Input: part model. Units: mm. Frame: model coordinates. A direction names the side the tool comes from. Give positions to 0.01 mm unless a question says otherwise; leave off trailing zeros. Order: outer loops, then holes, each group sorted by start corner. A loop starts at its lowest first (then second) coordinate and runs counter-clockwise, first axis right, second up.
```python
from build123d import *

# Parameters (mm, degrees)
SKETCH1_W           = 40
SKETCH1_H           = 40
BOSS_EXTRUDE1_DEPTH = 5
SKETCH3_W           = 5
SKETCH3_H           = 40
BOSS_EXTRUDE6_DEPTH = 40
SKETCH4_R           = 2.25
CUT_EXTRUDE2_DEPTH  = 49.989794856
SKETCH5_R           = 10.5
SKETCH5_R_2         = 2
CUT_EXTRUDE3_DEPTH  = 61.415229868


with BuildPart() as part:
    # Sketch1 → Boss-Extrude1 (new body)
    with BuildSketch(Plane(origin=(0, 0, 0), x_dir=(1, 0, 0), z_dir=(0, 1, 0))):
        Rectangle(SKETCH1_W, SKETCH1_H)
    extrude(amount=BOSS_EXTRUDE1_DEPTH)

    # Sketch3 → Boss-Extrude6 (add)
    with BuildSketch(Plane(origin=(0, 5, 0), x_dir=(1, 0, 0), z_dir=(0, 1, 0))):
        with Locations((-17.5, 0)):
            Rectangle(SKETCH3_W, SKETCH3_H)
    extrude(amount=BOSS_EXTRUDE6_DEPTH)

    # Sketch4 → Cut-Extrude2 (cut, through all)
    with BuildSketch(Plane(origin=(0, 5, 0), x_dir=(1, 0, 0), z_dir=(0, 1, 0))):
        with Locations(Location((10, 12, 0), (0, 0, 270))):
            Circle(SKETCH4_R)
        with Locations(Location((10, -12, 0), (0, 0, 90))):
            Circle(SKETCH4_R)
    extrude(amount=-CUT_EXTRUDE2_DEPTH, mode=Mode.SUBTRACT)

    # Sketch5 → Cut-Extrude3 (cut, through all)
    with BuildSketch(Plane(origin=(-15, 0, 0), x_dir=(0, 0, -1), z_dir=(1, 0, 0))):
        with Locations((0, 25)):
            Circle(SKETCH5_R)
        with Locations((-10.606601718, 35.606601718)):
            Circle(SKETCH5_R_2)
        with Locations((10.606601718, 35.606601718)):
            Circle(SKETCH5_R_2)
        with Locations((10.606601718, 14.393398282)):
            Circle(SKETCH5_R_2)
        with Locations((-10.606601718, 14.393398282)):
            Circle(SKETCH5_R_2)
    extrude(amount=-CUT_EXTRUDE3_DEPTH, mode=Mode.SUBTRACT)


solid = part.part
```
1) Cut plane D-D (z = 12). Return the cut outline in (x, y).
2) Line query: probe 1 along X at (y, z) = (3.1, -12); probe 2 along Y at (x, z) = (-16, -0.5); probe 3 along X at (y, z) = (7, -2). Output: solid intervals per line, ascending.
3) Cut plane C-C (y = 3). Return the cut outline in (x, z).
4) Reachability of faces 5 (the face through (11.52, 2.54, -13.66)), 6 (the face through (2, 5, 0)) from +Z, -Z, +X, -X, +Y, -Y: full face, straight path, thin tool, end or side. Return the list, or none.
5) Cut plane B-B (z = 0). Return the cut outline in (x, y).
6) Pull-direction query (Y, two-part tool) for faces 1 (the face through (-15, 16, -9)), 2 (the face through (-17.465, 14.994, -12.514)), 3 (the face through (0, 0, 0)), 4 (the face through (-17.465, 33.654, 11.04)); classes: pulls with the +Y half, pulls with the -Y half, needs draft (parallel to the pull), parting line crosses it, or undercut.
7) Cut plane A-A (y = 25). Return the cut outline in (x, z), then the cut area to 3 significant figures.
8) First-contact query: P1, Ø5, axis at y = 14.39, z = 10.61, coming from the +X side; P2, Ø4, axis at x = -1.5, z = -2.5, coming from the +Y side; P3, Ø3.5, axis at y = 35.61, z = -10.61, coming from the -X side. Flat tips, straight axial feed; report the tip coordinate or a pass-through.
Geometry says:
1. outline: (-20, 0) - (7.75, 0) - (7.75, 5) - (-15, 5) - (-15, 12.96) - (-20, 12.96) - close; (-20, 15.83) - (-15, 15.83) - (-15, 34.17) - (-20, 34.17) - close; (-20, 37.04) - (-15, 37.04) - (-15, 45) - (-20, 45) - close; (12.25, 0) - (20, 0) - (20, 5) - (12.25, 5) - close
2. probe 1: x = -20 to 7.75, 12.25 to 20
2. probe 2: y = 0 to 14.51, 35.49 to 45
2. probe 3: x = -20 to -15
3. outline: (-20, -20) - (20, -20) - (20, 20) - (-20, 20) - close; hole circle Ø4.5 at (10, -12); hole circle Ø4.5 at (10, 12)
4. face 5: +Y, -Y
4. face 6: +Z, -Z, +X, +Y
5. outline: (-20, 0) - (20, 0) - (20, 5) - (-15, 5) - (-15, 14.5) - (-20, 14.5) - close; (-20, 35.5) - (-15, 35.5) - (-15, 45) - (-20, 45) - close
6. face 1: needs draft
6. face 2: undercut
6. face 3: pulls with the -Y half
6. face 4: undercut
7. outline: (-20, -20) - (-15, -20) - (-15, -10.5) - (-20, -10.5) - close; (-20, 10.5) - (-15, 10.5) - (-15, 20) - (-20, 20) - close
7. area: 95.0 mm2
8. P1: stops at x = -15
8. P2: stops at y = 5
8. P3: passes through
